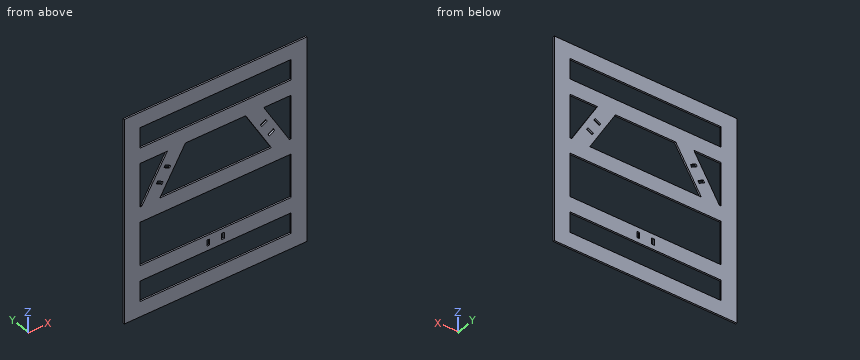
from build123d import *

# Parameters (mm, degrees)
CROQUIS1_W              = 350
CROQUIS1_H              = 400
CROQUIS1_W_2            = 290
CROQUIS1_H_2            = 340
CROQUIS1_H_3            = 30
SALIENTE_EXTRUIR1_DEPTH = 3
CROQUIS9_W              = 5.1
CROQUIS9_H              = 12.1
CORTAR_EXTRUIR3_DEPTH   = 4
MATRIZC2_COUNT          = 3


with BuildPart() as part:
    # Croquis1 → Saliente-Extruir1 (new body)
    with BuildSketch(Plane(origin=(0, 0, 0), x_dir=(1, 0, 0), z_dir=(0, 1, 0))):
        Rectangle(CROQUIS1_W, CROQUIS1_H)
        Rectangle(CROQUIS1_W_2, CROQUIS1_H_2, mode=Mode.SUBTRACT)
        with Locations((0, 115)):
            Rectangle(CROQUIS1_W_2, CROQUIS1_H_3)
        Polygon((-145, 15), (-145, -15), (-141.450815951, -15), (-106.8097998, -15), (106.8097998, -15), (141.450815951, -15), (145, -15), (145, 15), align=None)
        Polygon((-145, -100), (-145, -130), (145, -130), (145, -100), (92.37604307, -100), (57.735026919, -100), (-57.735026919, -100), (-92.37604307, -100), align=None)
        Polygon((-141.450815951, -15), (-92.37604307, -100), (-57.735026919, -100), (-106.8097998, -15), align=None)
        Polygon((57.735026919, -100), (92.37604307, -100), (141.450815951, -15), (106.8097998, -15), align=None)
    extrude(amount=SALIENTE_EXTRUIR1_DEPTH)

    # Croquis9 → Cortar-Extruir3 (cut, through all)
    with BuildSketch(Plane(origin=(0, 0, 0), x_dir=(1, 0, 0), z_dir=(0, 1, 0))):
        with Locations((-14.35, 115)):
            Rectangle(CROQUIS9_W, CROQUIS9_H)
        with Locations((14.35, 115)):
            Rectangle(CROQUIS9_W, CROQUIS9_H)
    cortar_extruir3 = extrude(amount=CORTAR_EXTRUIR3_DEPTH, mode=Mode.SUBTRACT)

    # MatrizC2: Cortar-Extruir3 ×3 about axis
    matrizc2_axis = Axis((0, 0, 0), (0, 1, 0))
    for i in range(1, MATRIZC2_COUNT):
        add(cortar_extruir3.rotate(matrizc2_axis, i * 360 / MATRIZC2_COUNT), mode=Mode.SUBTRACT)


solid = part.part
Geometry check sheet. Reference: the model listing, model coordinates, mm. Round coordinates to 2 decimals unless told otherwise and drop trailing zeros. Loops run counter-clockwise (first coordinate to the right, second up) from the corner with the lowest first, then second, coordinate; pieces in that order, holes last. Notation, with made-up numbers: (-13, 81.5) -> (14, 81.5) arc R28 cw to (14, 119.5) -> close; hole circle Ø3 at (35.25, -30.5). An arc over 180 degrees is marked (long way). Answer as a JSON object with one key per item and string values. Group by question number.
Item 1: Cross-section at D-D, the plane y = 1.6. Count the separate pieces of the cut face and the enclosed holes in it, plus the area to 3 significant figures.
Item 2: Thickness scan on line 1 along X through (y, z) = (0.65, -116); line 2 along Z through (x, y) = (-36.5, 2.05); line 3 along X through (y, z) = (0.35, -136). Record the ranges inside material, lowest first.
Item 3: Cross-section at A-A, the plane x = -36. Record the cut outline in (y, z).
Item 4: Cross-section at B-B, the plane z = -156. Record the cut outline in (x, y), plus the area to 3 significant figures.
Item 5: Cross-section at C-C, the plane z = -116. Record the cut outline in (x, y), plus the area to 3 significant figures.
Determined:
{
 "1": {"separate pieces": "1", "enclosed holes": "12", "area": "73,000 mm²"},
 "2": {"line 1": "x = -175 to -16.9, -11.8 to 11.8, 16.9 to 175", "line 2": "z = -200 to -170, -130 to -100, -15 to 15, 100 to 130, 170 to 200", "line 3": "x = -175 to -145, 145 to 175"},
 "3": {"outline": "(0, -200) -> (3, -200) -> (3, -170) -> (0, -170) -> close; (0, -130) -> (3, -130) -> (3, -100) -> (0, -100) -> close; (0, -15) -> (3, -15) -> (3, 15) -> (0, 15) -> close; (0, 100) -> (3, 100) -> (3, 130) -> (0, 130) -> close; (0, 170) -> (3, 170) -> (3, 200) -> (0, 200) -> close"},
 "4": {"outline": "(-175, 0) -> (-145, 0) -> (-145, 3) -> (-175, 3) -> close; (145, 0) -> (175, 0) -> (175, 3) -> (145, 3) -> close", "area": "180 mm²"},
 "5": {"outline": "(-175, 0) -> (-16.9, 0) -> (-16.9, 3) -> (-175, 3) -> close; (-11.8, 0) -> (11.8, 0) -> (11.8, 3) -> (-11.8, 3) -> close; (16.9, 0) -> (175, 0) -> (175, 3) -> (16.9, 3) -> close", "area": "1,020 mm²"}
}
